```python
from build123d import *

# Parameters (mm, degrees)
BOSS_EXTRUDE1_DEPTH = 20
BOSS_EXTRUDE2_DEPTH = 10
CUT_EXTRUDE1_DEPTH  = 20


with BuildPart() as part:
    # Sketch1 → Boss-Extrude1 (new body, symmetric)
    with BuildSketch(Plane.XY):
        with BuildLine():
            Line((0, 0), (100, 0))
            Line((100, 0), (75, 30))
            Line((75, 30), (40, 30))
            Line((40, 30), (40, 45))
            ThreePointArc((40, 45), (34.142135624, 59.142135624), (20, 65))
            ThreePointArc((20, 65), (5.857864376, 59.142135624), (0, 45))
            Line((0, 45), (0, 0))
        make_face()
    extrude(amount=BOSS_EXTRUDE1_DEPTH, both=True)

    # Sketch2 → Boss-Extrude2 (add, symmetric)
    with BuildSketch(Plane.XY):
        Polygon((40, 30), (40, 45), (64.995844506, 45), (75, 30), align=None)
    extrude(amount=BOSS_EXTRUDE2_DEPTH, both=True)

    # Sketch3 → Cut-Extrude1 (cut, symmetric)
    with BuildSketch(Plane.XY):
        with BuildLine():
            Line((10, 0), (10, 45))
            ThreePointArc((10, 45), (20, 55), (30, 45))
            Line((30, 45), (30, 0))
            Line((30, 0), (10, 0))
        make_face()
    extrude(amount=CUT_EXTRUDE1_DEPTH, both=True, mode=Mode.SUBTRACT)


solid = part.part
```
Input: part model. Units: mm. Frame: model coordinates. A direction names the side the tool comes from. Round coordinates to 2 decimals unless told otherwise and drop trailing zeros. Loops run counter-clockwise (first coordinate to the right, second up) from the corner with the lowest first, then second, coordinate; pieces in that order, holes last.
1) Section query B-B on z = -16.5. Return the cut outline in (x, y), plus the area to 3 significant figures.
Ans:
outline: (0, 0) - (10, 0) - (10, 45) arc R10 cw to (30, 45) - (30, 0) - (100, 0) - (75, 30) - (40, 30) - (40, 45) arc R20 ccw to (0, 45) - close
area: 2,800 mm2
2) Section query A-A on y = 18. Return the cut outline in (x, z), plus the area to 3 significant figures.
Ans:
outline: (0, -20) - (10, -20) - (10, 20) - (0, 20) - close; (30, -20) - (85, -20) - (85, 20) - (30, 20) - close
area: 2,600 mm2
3) Pin query (flat end, axial travel): pin 1 (16 mm diameter, centred on x = 46.5, z = -3, fed in from +Y); pin 2 (4 mm diameter, centred on y = 54.5, z = 4.5, fed in from +X); pin 3 (7.5 mm diameter, centred on x = 56, y = 35.5, fed in from -Z); pin 4 (1 mm diameter, centred on x = 48, z = -2.5, fed in from -Y). Return the tip coordinate at first contact, or that it passes through.
Ans:
pin 1: stops at y = 52.6
pin 2: stops at x = 38.54
pin 3: stops at z = -10
pin 4: stops at y = 0
4) Pull-direction query (X, two-part tool) for faces 5 (the flat face through (10, 22, 0)), 6 (the flat face through (54, 38, -10)), 7 (the flat face through (87.675, 14.79, 0.28)); classes: released by +X, released by -X, zero draft, split by the parting line, or undercut.
Ans:
face 5: undercut
face 6: zero draft
face 7: released by +X
5) Section query C-C on x = 46. Return the cut outline in (y, z).
Ans:
outline: (0, -20) - (30, -20) - (30, -10) - (45, -10) - (45, 10) - (30, 10) - (30, 20) - (0, 20) - close
6) Section query D-D on y = 31.5. Return the cut outline in (x, z).
Ans:
outline: (0, -20) - (10, -20) - (10, 20) - (0, 20) - close; (30, -20) - (40, -20) - (40, -10) - (74, -10) - (74, 10) - (40, 10) - (40, 20) - (30, 20) - close
7) Set-up query: faces 1 (the flat face through (52, 45, 0)), 2 (the flat face through (58, 30, -15)), 3 (the flat face through (40, 37, 15)), 4 (the flat face through (30, 23, 0)). Return all of +Z, -Z, +X, -X, +Y, -Y with unobstructed straight access to the full face (end or side cutting, diameter ignored); none if empty.
Ans:
face 1: +Z, -Z, +X, +Y
face 2: -Z, +X, +Y
face 3: +Z, +X, +Y
face 4: +Z, -Z, -Y
8) Material intervals for line 1 (X direction, y = 40.5, z = -13); line 2 (Y direction, x = 52, z = -11); line 3 (X direction, y = 27, z = -17), sorted ascending.
Ans:
line 1: x = 0 to 10, 30 to 40
line 2: y = 0 to 30
line 3: x = 0 to 10, 30 to 77.5
